from build123d import *

# Parameters (mm, degrees)
EXTRUDE1_DEPTH     = 28.702
SKETCH3_OUTSIDE_W  = 244.651
SKETCH3_OUTSIDE_H  = 249.072
SKETCH3_OUTSIDE_R  = 14.2875
CUT_EXTRUDE1_DEPTH = 37.057098264
CUT_EXTRUDE1_DRAFT = -70
SKETCH4_OUTSIDE_W  = 244.652
SKETCH4_OUTSIDE_H  = 249.072
SKETCH4_OUTSIDE_R  = 14.2875
CUT_EXTRUDE2_DEPTH = 37.057098264
CUT_EXTRUDE2_DRAFT = -70
SKETCH5_R          = 8.5725
EXTRUDE2_DEPTH     = 14.224
EXTRUDE2_DRAFT     = 1.5
SKETCH7_R          = 10.668
CUT_EXTRUDE4_DEPTH = 37.591086429
CUT_EXTRUDE4_DRAFT = 1.5
SKETCH12_W         = 6.35
SKETCH12_H         = 16.497783942
SKETCH15_R         = 11.276975829
CUT_EXTRUDE7_DEPTH = 5.08
CUT_EXTRUDE7_DRAFT = -45


with BuildPart() as part:
    # Sketch2 → Extrude1 (new body)
    with BuildSketch(Plane(origin=(-21.463, 0, 0), x_dir=(0, 0, -1), z_dir=(1, 0, 0))):
        Polygon((0, 16.497783942), (-14.2875, 8.248891971), (-14.2875, -8.248891971), (0, -16.497783942), (14.2875, -8.248891971), (14.2875, 8.248891971), align=None)
    extrude(amount=EXTRUDE1_DEPTH)


with BuildPart() as cut_extrude1_tool:
    # Sketch3 outside → Cut-Extrude1 (with draft: the straight prism first)
    with BuildSketch(Plane(origin=(7.239, 0, 0), x_dir=(0, 0, -1), z_dir=(1, 0, 0))):
        with Locations((-0.0005, 0)):
            Rectangle(SKETCH3_OUTSIDE_W, SKETCH3_OUTSIDE_H)
        Circle(SKETCH3_OUTSIDE_R, mode=Mode.SUBTRACT)
    extrude(amount=-CUT_EXTRUDE1_DEPTH)
    # Cut-Extrude1: the draft: its side faces are tilted about the plane it starts from
    cut_extrude1_sides = [cut_extrude1_tool.faces().sort_by_distance(p)[0] for p in [
        (-11.289549132, -124.536, 0.0005),
        (-11.289549132, 0, -122.325),
        (-11.289549132, 124.536, 0.0005),
        (-11.289549132, 0, 122.326),
        (-11.289549132, 0, 14.2875),
    ]]
    draft(cut_extrude1_sides, Plane(origin=(7.239, 0, 0), x_dir=(0, 0, -1), z_dir=(1, 0, 0)), CUT_EXTRUDE1_DRAFT)


with BuildPart() as part_1:
    add(part.part)

    # Cut-Extrude1: cut by cut_extrude1_tool
    add(cut_extrude1_tool.part, mode=Mode.SUBTRACT)


with BuildPart() as cut_extrude2_tool:
    # Sketch4 outside → Cut-Extrude2 (with draft: the straight prism first)
    with BuildSketch(Plane.ZY.offset(21.463)):
        Rectangle(SKETCH4_OUTSIDE_W, SKETCH4_OUTSIDE_H)
        Circle(SKETCH4_OUTSIDE_R, mode=Mode.SUBTRACT)
    extrude(amount=-CUT_EXTRUDE2_DEPTH)
    # Cut-Extrude2: the draft: its side faces are tilted about the plane it starts from
    cut_extrude2_sides = [cut_extrude2_tool.faces().sort_by_distance(p)[0] for p in [
        (-2.934450868, -124.536, 0),
        (-2.934450868, 0, 122.326),
        (-2.934450868, 124.536, 0),
        (-2.934450868, 0, -122.326),
        (-2.934450868, 0, -14.2875),
    ]]
    draft(cut_extrude2_sides, Plane.ZY.offset(21.463), CUT_EXTRUDE2_DRAFT)


with BuildPart() as part_2:
    add(part_1.part)

    # Cut-Extrude2: cut by cut_extrude2_tool
    add(cut_extrude2_tool.part, mode=Mode.SUBTRACT)


with BuildPart() as body_2:
    # Sketch5 → Extrude2 (with draft: the straight prism first)
    with BuildSketch(Plane(origin=(21.463, 0, 0), x_dir=(0, 0, -1), z_dir=(1, 0, 0))):
        Circle(SKETCH5_R)
    extrude(amount=-EXTRUDE2_DEPTH)
    # Extrude2: the draft: its side faces are tilted about the plane it starts from
    extrude2_sides = [body_2.faces().sort_by_distance(p)[0] for p in [
        (14.351, 0, 8.5725),
    ]]
    draft(extrude2_sides, Plane(origin=(21.463, 0, 0), x_dir=(0, 0, -1), z_dir=(1, 0, 0)), EXTRUDE2_DRAFT)

    # Sketch17 → Cut-Revolve2 (revolve, cut)
    with BuildSketch(Plane.XY, mode=Mode.PRIVATE) as cut_revolve2_sk:
        Polygon((21.463, 8.814890815), (21.463, 7.274956448), (19.923065632, 8.814890815), align=None)
        Polygon((7.239, 7.893804996), (8.226777778, 7.893804996), (9.528863597, 9.195890815), (7.239, 9.195890815), align=None)
    revolve(cut_revolve2_sk.sketch.rotate(Axis((-21.463, 0, 0), (1, 0, 0)), 270), axis=Axis((-21.463, 0, 0), (1, 0, 0)), mode=Mode.SUBTRACT)


with BuildPart() as cut_extrude4_tool:
    # Sketch7 → Cut-Extrude4 (with draft: the straight prism first)
    with BuildSketch(Plane(origin=(-7.90702, 0, 0), x_dir=(0, 0, -1), z_dir=(1, 0, 0))):
        Circle(SKETCH7_R)
    extrude(amount=-CUT_EXTRUDE4_DEPTH)
    # Cut-Extrude4: the draft: its side faces are tilted about the plane it starts from
    cut_extrude4_sides = [cut_extrude4_tool.faces().sort_by_distance(p)[0] for p in [
        (-26.702563214, 0, 10.668),
    ]]
    draft(cut_extrude4_sides, Plane(origin=(-7.90702, 0, 0), x_dir=(0, 0, -1), z_dir=(1, 0, 0)), CUT_EXTRUDE4_DRAFT)


with BuildPart() as part_3:
    add(part_2.part)

    # Cut-Extrude4: cut by cut_extrude4_tool
    add(cut_extrude4_tool.part, mode=Mode.SUBTRACT)


with BuildPart() as body_2_1:
    add(body_2.part)

    # Combine1: union part
    add(part_3.part)

    # Sketch12 → Cut-Revolve1 (revolve, cut)
    with BuildSketch(Plane.XY, mode=Mode.PRIVATE) as cut_revolve1_sk:
        Polygon((-7.90702, 10.078793431), (-7.90702, 0), (21.463, 0), (21.463, 5.207), (-3.035226569, 5.207), align=None)
        with Locations((-24.638, 8.248891971)):
            Rectangle(SKETCH12_W, SKETCH12_H)
    revolve(cut_revolve1_sk.sketch.rotate(Axis((-21.463, 0, 0), (1, 0, 0)), 90), axis=Axis((-21.463, 0, 0), (1, 0, 0)), mode=Mode.SUBTRACT)


with BuildPart() as cut_extrude7_tool:
    # Sketch15 → Cut-Extrude7 (with draft: the straight prism first)
    with BuildSketch(Plane.ZY.offset(21.463)):
        Circle(SKETCH15_R)
    extrude(amount=-CUT_EXTRUDE7_DEPTH)
    # Cut-Extrude7: the draft: its side faces are tilted about the plane it starts from
    cut_extrude7_sides = [cut_extrude7_tool.faces().sort_by_distance(p)[0] for p in [
        (-18.923, 0, -11.276975829),
    ]]
    draft(cut_extrude7_sides, Plane.ZY.offset(21.463), CUT_EXTRUDE7_DRAFT)


with BuildPart() as body_2_2:
    add(body_2_1.part)

    # Cut-Extrude7: cut by cut_extrude7_tool
    add(cut_extrude7_tool.part, mode=Mode.SUBTRACT)


solid = body_2_2.part
Work out the finished part from the listing and answer in its coordinate system (mm). A direction names the side the tool comes from. Round coordinates to 2 decimals unless told otherwise and drop trailing zeros. Loops run counter-clockwise (first coordinate to the right, second up) from the corner with the lowest first, then second, coordinate; pieces in that order, holes last. Notation, with made-up numbers: M 47,33.25 L 60,33.25 A16 cw 60,51.25 Z; hole C 48,24.5 d5. An arc over 180 degrees is marked long. One line per question, with ' | ' between items. Start each with the question number.
(1) Flat-ended cylindrical pins translate along their axes: pin 1 Ø2 at (x, z) = (3.5, -2.5) entering from -Y; pin 2 Ø1 at (y, z) = (-6, 4) entering from -X; pin 3 Ø2 at (x, z) = (2.5, -3) entering from -Y; pin 4 Ø5 at (y, z) = (-12.5, -9.5) entering from -X. Find the tip coordinate at first contact, or state that the pin passes through.
(2) A cutting plane is placed at A-A on x = 15.5. Write down the section's boundary in (y, z).
(3) For a pull along X with two mould halves and no side action, classify faces 1 (the face through (14.755, 2.628, -8.344)), 2 (the face through (7.74, -4.803, 6.264)), 3 (the face through (-21.27, -7.38, -12.85)) as released by +X, released by -X, zero draft, split by the parting line, or undercut.
(4) Find the intervals of material crossed by line 1 (Y direction, x = 3.75, z = 0); line 2 (Z direction, x = -10.5, y = -6); line 3 (X direction, y = 5, z = -6.75), in increasing order.
(5) A tool of negligible diameter and unlimited length cuts with its end or side. For faces 4 (the face through (21.463, 2, 5)), 5 (the face through (-7.907, -9, -5)), from which of +Z, -Z, +X, -X, +Y, -Y can it reach the whole face along a straight path? Write none if from no direction.
Geometry check:
1) pin 1: stops at y = -15.63 | pin 2: stops at x = -5.54 | pin 3: stops at y = -15.34 | pin 4: stops at x = -21.46
2) outline: C 0,0 d17.46; hole C 0,0 d10.41
3) face 1: released by +X | face 2: undercut | face 3: released by -X
4) line 1: y = -16.5 to -5.21, 5.21 to 16.5 | line 2: z = -14.29 to -8.9, 8.9 to 14.29 | line 3: x = -6.23 to 7.24, 8.73 to 20.34
5) face 4: +Z, -Z, +X, +Y, -Y | face 5: -X
